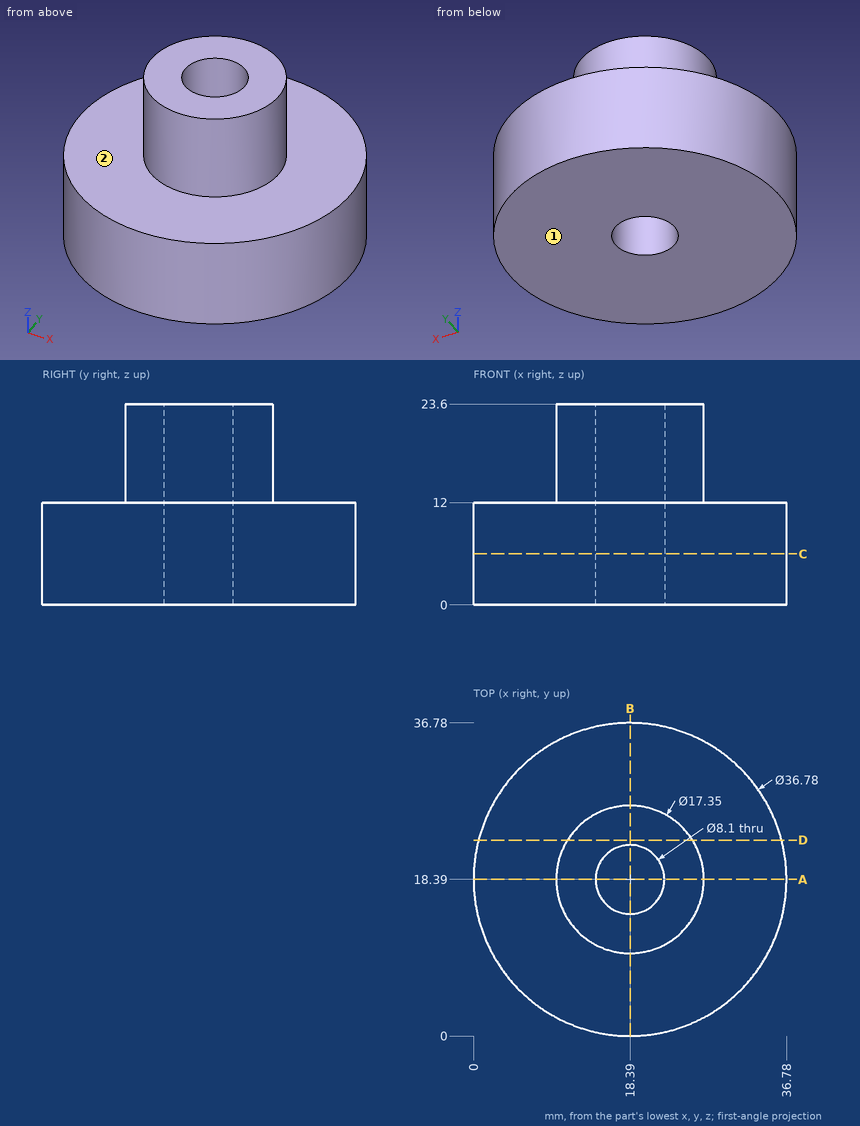
Print and shaded views of the part. All mm, measured from the part's lowest x, y and z. A direction names the side the tool comes from. Round coordinates to 2 decimals unless told otherwise and drop trailing zeros. Write each loop counter-clockwise with the first axis right and the second up, starting at its lowest first coordinate (ties: lowest second). Pieces come first, ordered by that corner, then holes. Notation, with made-up numbers: M 59,59 L 87,59 A18 cw 87,65 Z; hole C 35,74.25 d4. An arc over 180 degrees is marked long. Use a Markdown table: item, result. Add a question column.
1. Slice it at A-A on y = 18.39. Give the cut face in (x, z) (3 decimals).
2. 3-axis set-ups, long thin cutter, end or side, ignore diameter. For the marked faces 1 and 2: which of +Z, -Z, +X, -X, +Y, -Y reach the whole face in a straight line?
3. Slice it at C-C on z = 6. Give the cut face in (x, y), then the cut area to 3 significant figures.
4. Slice it at D-D on y = 23. Give the cut face in (x, z), then the cut area to 3 significant figures.
5. Flat gauge pins, fed straight in: P1, Ø9.5, axis at x = 18.39, y = 18.39, coming from the +Z side; P2, Ø10, axis at x = 13, z = 5, coming from the +Y side; P3, Ø8, axis at x = 15, y = 31.5, coming from the +Z side; P4, Ø1.5, axis at y = 14, z = 8, coming from the +X side. Where does each tip first touch, or does it go through?
6. Drill centre lines: probe 1 along Y at (x, z) = (18.39, 5.5); probe 2 along Y at (x, z) = (18.39, 15) (3 decimals); probe 3 along Z at (x, y) = (10.5, 28). Where is each one in solid material? Low to high.
Reply:
| question | item | result |
|---|---|---|
| 1 | outline | M 0,0 L 14.34,0 L 14.34,23.6 L 9.715,23.6 L 9.715,12 L 0,12 Z; M 22.44,0 L 36.78,0 L 36.78,12 L 27.065,12 L 27.065,23.6 L 22.44,23.6 Z |
| 2 | face 1 | -Z, +X, -X, +Y, -Y |
| 2 | face 2 | +Z |
| 3 | outline | C 18.39,18.39 d36.78; hole C 18.39,18.39 d8.1 |
| 3 | area | 1,010 mm^2 |
| 4 | outline | M 0.59,0 L 36.19,0 L 36.19,12 L 25.74,12 L 25.74,23.6 L 11.04,23.6 L 11.04,12 L 0.59,12 Z |
| 4 | area | 598 mm^2 |
| 5 | P1 | stops at z = 23.6 |
| 5 | P2 | stops at y = 36.78 |
| 5 | P3 | stops at z = 12 |
| 5 | P4 | stops at x = 36.42 |
| 6 | probe 1 | y = 0 to 14.34, 22.44 to 36.78 |
| 6 | probe 2 | y = 9.715 to 14.34, 22.44 to 27.065 |
| 6 | probe 3 | z = 0 to 12 |
